Design review of the part built by this model. Coordinates are the model's own, in mm. A direction names the side the tool comes from. Round coordinates to 2 decimals unless told otherwise and drop trailing zeros. Order: outer loops, then holes, each group sorted by start corner. A loop starts at its lowest first (then second) coordinate and runs counter-clockwise, first axis right, second up. Notation, with made-up numbers: (68.25, -30.5) - (80.25, -30.5) arc R31 ccw to (80.25, 0.5) - close; hole circle Ø6 at (53, 10.5). An arc over 180 degrees is marked (long way). Answer as a JSON object with one key per item and string values. Group by question number.
from build123d import *

# Parameters (mm, degrees)
SKETCH105_W     = 55
SKETCH105_H     = 56
PAD075_DEPTH    = 18
SKETCH012_W     = 52.6
SKETCH012_H     = 53.6
POCKET028_DEPTH = 16.8
POCKET029_DEPTH = 1.2
SKETCH014_W     = 17
SKETCH014_H     = 3.5
POCKET030_DEPTH = 1.2
SKETCH015_R     = 2.5
SKETCH015_R_2   = 0.9
PAD010_DEPTH    = 2.5


with BuildPart() as part:
    # Sketch105 → Pad075 (new body)
    with BuildSketch(Plane.XY):
        Rectangle(SKETCH105_W, SKETCH105_H)
    extrude(amount=PAD075_DEPTH)

    # Sketch012 (on Face6 of Pad075) → Pocket028 (cut)
    with BuildSketch(Plane.XY.offset(18)):
        Rectangle(SKETCH012_W, SKETCH012_H)
    extrude(amount=-POCKET028_DEPTH, mode=Mode.SUBTRACT)

    # Sketch013 (on Face6 of Pocket028) → Pocket029 (cut)
    with BuildSketch(Plane.XZ.offset(28)):
        with BuildLine():
            ThreePointArc((12.47, 9.000073), (15.239982, 11.74), (12.49, 14.5))
            Line((9.66, 14.5), (12.49, 14.5))
            Line((9.66, 14.5), (9.962666, 15.767791))
            ThreePointArc((9.962666, 15.767791), (9.774923, 16.619593), (8.99, 17))
            Line((-9.01, 17), (8.99, 17))
            ThreePointArc((-9.01, 17), (-9.794923, 16.619593), (-9.982666, 15.767791))
            Line((-9.68, 14.5), (-9.982666, 15.767791))
            Line((-12.51, 14.5), (-9.68, 14.5))
            ThreePointArc((-12.51, 14.5), (-15.26, 11.75), (-12.51, 9))
            Line((-12.51, 9), (-8.39, 9))
            Line((-7.983449, 7.271094), (-8.39, 9))
            ThreePointArc((-7.983449, 7.271094), (-7.630924, 6.716129), (-7.01, 6.5))
            Line((6.99, 6.5), (-7.01, 6.5))
            ThreePointArc((6.99, 6.5), (7.615236, 6.719564), (7.965913, 7.281839))
            Line((7.965913, 7.281839), (8.35, 9))
            Line((8.35, 9), (12.47, 9.000073))
        make_face()
    extrude(amount=-POCKET029_DEPTH, mode=Mode.SUBTRACT)

    # Sketch014 (on Face2 of Pocket029) → Pocket030 (cut)
    with BuildSketch(Plane(origin=(-27.5, 0, 0), x_dir=(0, -1, 0), z_dir=(-1, 0, 0))):
        with Locations((2.6, 6.75)):
            Rectangle(SKETCH014_W, SKETCH014_H)
    extrude(amount=-POCKET030_DEPTH, mode=Mode.SUBTRACT)

    # Sketch015 (on Face31 of Pocket030) → Pad010 (join)
    with BuildSketch(Plane.XY.offset(1.2)):
        with Locations((22, -23.05)):
            Circle(SKETCH015_R)
        with Locations((22, -23.05)):
            Circle(SKETCH015_R_2, mode=Mode.SUBTRACT)
        with Locations((-22, -23.05)):
            Circle(SKETCH015_R)
        with Locations((-22, -23.05)):
            Circle(SKETCH015_R_2, mode=Mode.SUBTRACT)
        with Locations((22, 20.95)):
            Circle(SKETCH015_R)
        with Locations((22, 20.95)):
            Circle(SKETCH015_R_2, mode=Mode.SUBTRACT)
        with Locations((-22, 20.95)):
            Circle(SKETCH015_R)
        with Locations((-22, 20.95)):
            Circle(SKETCH015_R_2, mode=Mode.SUBTRACT)
    extrude(amount=PAD010_DEPTH)


solid = part.part
1. Clearance check with flat-ended pins moving along their axes: P1, Ø1.4, axis at x = 22, y = -23.05, coming from the +Z side; P2, Ø0.6, axis at x = -1.5, y = -27.5, coming from the -Z side; P3, Ø2.5, axis at x = 21.5, y = -23.5, coming from the +Z side. State where each tip first meets the part, or that it passes through.
2. Take a section at A-A, the plane x = 4.5. Give the boundary of the cut face in (y, z).
3. Take a section at B-B, the plane z = 11.75. Give the boundary of the cut face in (x, y).
4. To check wall thickness, follow line 1 (Y direction, x = 22, z = 3.25); line 2 (Y direction, x = 1, z = 2.5); line 3 (X direction, y = 1, z = 12.75). State the ranges of each line that lie inside material, in increasing order. Write a range as from..to.
5. Take a section at D-D, the plane x = -18.5. Give the boundary of the cut face in (y, z), then the cut area to 3 significant figures.
6. Take a section at C-C, the plane y = -9. Give the boundary of the cut face in (x, z), then the cut area to 3 significant figures.
7. Mouldability with a two-part tool opening along X and no side actions: class faces 1 (the flat face through (0, 28, 9)), 2 (the flat face through (-20.9, 21, 3.7)), 3 (the cylindrical face through (22.415, 20.152, 2.432)) as pulls with the +X half, pulls with the -X half, needs draft (parallel to the pull), parting line crosses it, or undercut.
8. Tool access review of faces 4 (the cylindrical face through (15.24, -27.41, 11.68)), 5 (the flat face through (22, -23, 1.2)), 6 (the flat face through (-27, 0, 18)): name each direction out of +Z, -Z, +X, -X, +Y, -Y from which nothing blocks a thin tool from reaching the whole face with its end or side.
Response values:
{
 "1": {"P1": "z = 1.2", "P2": "z = 0", "P3": "z = 3.7"},
 "2": {"outline": "(-28, 0) - (28, 0) - (28, 18) - (26.8, 18) - (26.8, 1.2) - (-26.8, 1.2) - (-26.8, 6.5) - (-28, 6.5) - close; (-28, 17) - (-26.8, 17) - (-26.8, 18) - (-28, 18) - close"},
 "3": {"outline": "(-27.5, -28) - (-15.26, -28) - (-15.26, -26.8) - (-26.3, -26.8) - (-26.3, 26.8) - (26.3, 26.8) - (26.3, -26.8) - (15.24, -26.8) - (15.24, -28) - (27.5, -28) - (27.5, 28) - (-27.5, 28) - close"},
 "4": {"line 1": "-28..-26.8, -25.55..-23.95, -22.15..-20.55, 18.45..20.05, 21.85..23.45, 26.8..28", "line 2": "-28..-26.8, 26.8..28", "line 3": "-27.5..-26.3, 26.3..27.5"},
 "5": {"outline": "(-28, 0) - (28, 0) - (28, 18) - (26.8, 18) - (26.8, 1.2) - (-26.8, 1.2) - (-26.8, 18) - (-28, 18) - close", "area": "108 mm2"},
 "6": {"outline": "(-27.5, 0) - (27.5, 0) - (27.5, 18) - (26.3, 18) - (26.3, 1.2) - (-26.3, 1.2) - (-26.3, 5) - (-27.5, 5) - close; (-27.5, 8.5) - (-26.3, 8.5) - (-26.3, 18) - (-27.5, 18) - close", "area": "102 mm2"},
 "7": {"face 1": "needs draft", "face 2": "undercut", "face 3": "undercut"},
 "8": {"face 4": "-Y", "face 5": "+Z", "face 6": "+Z, +X, -X, +Y, -Y"}
}
